from build123d import *

# Parameters (mm, degrees)
F0_W     = 43.3
F0_H     = 33.3
F0_W_2   = 40
F0_H_2   = 30
F1_DEPTH = 15
F2_DEPTH = 1.5
F3_W     = 41.6
F3_H     = 31.6
F3_W_2   = 40
F3_H_2   = 30
F4_DEPTH = 1
F5_R     = 1.3


with BuildPart() as f1:
    # F0 (on Top) → F1 (new body)
    with BuildSketch(Plane.XY):
        Rectangle(F0_W, F0_H)
        Rectangle(F0_W_2, F0_H_2, mode=Mode.SUBTRACT)
    extrude(amount=F1_DEPTH)

    # F0 (on Top) → F2 (join)
    with BuildSketch(Plane.XY):
        Rectangle(F0_W_2, F0_H_2)
    extrude(amount=F2_DEPTH)

    # F3 (on face) → F4 (join)
    with BuildSketch(Plane.XY.offset(15)):
        Rectangle(F3_W, F3_H)
        Rectangle(F3_W_2, F3_H_2, mode=Mode.SUBTRACT)
    extrude(amount=F4_DEPTH)

    # F5
    f5_edges = [f1.edges().sort_by_distance(p)[0] for p in [
        (-21.65, -16.65, 7.5),
        (21.65, -16.65, 7.5),
        (21.65, 16.65, 7.5),
        (-21.65, 16.65, 7.5),
    ]]
    fillet(f5_edges, radius=F5_R)


solid = f1.part
Geometry: final body of the model. Coordinates: model frame, mm. A direction names the side the tool comes from. Give positions to 0.01 mm unless a question says otherwise; leave off trailing zeros. Write each loop counter-clockwise with the first axis right and the second up, starting at its lowest first coordinate (ties: lowest second). Pieces come first, ordered by that corner, then holes. Notation, with made-up numbers: (57.5, 16) - (107.5, 16) arc R12 ccw to (107.5, 34) - close; hole circle Ø9 at (-9, -38.5). An arc over 180 degrees is marked (long way). Return JSON: item names as keys, results as strings. Group by question number.
1) Mould query, pull axis Y, two halves, no side actions, for faces 4 (the flat face through (20, 0, 9)), 5 (the flat face through (-0.3, -15.8, 15.5)), 6 (the flat face through (20.8, -0.2, 15.5)). Classes: released by +Y, released by -Y, zero draft, split by the parting line, or undercut.
2) Section A-A on z = 9.5. Return the cut outline in (x, y).
3) Set-up query: faces 1 (the flat face through (-20.8, -0.2, 15.5)), 2 (the flat face through (-0.3, 15.8, 15.5)), 3 (the flat face through (-20, 0, 9)). Return all of +Z, -Z, +X, -X, +Y, -Y with unobstructed straight access to the full face (end or side cutting, diameter ignored); none if empty.
4) Section B-B on x = 12. Return the cut outline in (y, z).
5) Line query: line 1 (Y direction, x = 14.5, z = 1.75); line 2 (X direction, y = -12.5, z = 9.5); line 3 (Z direction, x = 2.5, y = -9.5). Output: solid intervals per line, ascending.
6) Section C-C on y = -1.5. Return the cut outline in (x, z), plus the area to 3 significant figures.
7) First-contact query: P1, Ø4, axis at x = 14, y = -8.5, coming from the +Z side; P2, Ø0.8, axis at x = 5, z = 15.5, coming from the -Y side; P3, Ø8, axis at x = -16, y = 11.5, coming from the -Z side; P4, Ø0.8, axis at y = 6.5, z = 15.5, coming from the +X side. Flat tips, straight axial feed; report the tip coordinate or a pass-through.
Filled in:
{
 "1": {"face 4": "undercut", "face 5": "released by -Y", "face 6": "zero draft"},
 "2": {"outline": "(-21.65, -15.35) arc R1.3 ccw to (-20.35, -16.65) - (20.35, -16.65) arc R1.3 ccw to (21.65, -15.35) - (21.65, 15.35) arc R1.3 ccw to (20.35, 16.65) - (-20.35, 16.65) arc R1.3 ccw to (-21.65, 15.35) - close; hole (-20, -15) - (20, -15) - (20, 15) - (-20, 15) - close"},
 "3": {"face 1": "+Z, -X, +Y, -Y", "face 2": "+Z, +X, -X, +Y", "face 3": "+Z"},
 "4": {"outline": "(-16.65, 0) - (16.65, 0) - (16.65, 15) - (15.8, 15) - (15.8, 16) - (15, 16) - (15, 1.5) - (-15, 1.5) - (-15, 16) - (-15.8, 16) - (-15.8, 15) - (-16.65, 15) - close"},
 "5": {"line 1": "y = -16.65 to -15, 15 to 16.65", "line 2": "x = -21.65 to -20, 20 to 21.65", "line 3": "z = 0 to 1.5"},
 "6": {"outline": "(-21.65, 0) - (21.65, 0) - (21.65, 15) - (20.8, 15) - (20.8, 16) - (20, 16) - (20, 1.5) - (-20, 1.5) - (-20, 16) - (-20.8, 16) - (-20.8, 15) - (-21.65, 15) - close", "area": "111 mm^2"},
 "7": {"P1": "stops at z = 1.5", "P2": "stops at y = -15.8", "P3": "stops at z = 0", "P4": "stops at x = 20.8"}
}
